```python
from build123d import *

# Parameters (mm, degrees)
SKETCH2_W           = 230
SKETCH2_H           = 200
BOSS_EXTRUDE1_DEPTH = 180
CUT_EXTRUDE1_DEPTH  = 200
FILLET2_R           = 40
SKETCH4_R           = 30
CUT_EXTRUDE2_DEPTH  = 48
SKETCH5_W           = 80
SKETCH5_H           = 129.575317766
CUT_EXTRUDE3_DEPTH  = 180
SKETCH6_R           = 15
CUT_EXTRUDE5_DEPTH  = 200


with BuildPart() as part:
    # Sketch2 → Boss-Extrude1 (new body)
    with BuildSketch(Plane(origin=(0, 0, 0), x_dir=(1, 0, 0), z_dir=(0, 1, 0))):
        with Locations((71.865714122, -63.208991457)):
            Rectangle(SKETCH2_W, SKETCH2_H)
    extrude(amount=BOSS_EXTRUDE1_DEPTH)

    # Sketch3 → Cut-Extrude1 (cut)
    with BuildSketch(Plane.XY.offset(163.208991457)):
        Polygon((100.422581047, 180), (186.865714122, 180), (186.865714122, 50.424682234), align=None)
    extrude(amount=-CUT_EXTRUDE1_DEPTH, mode=Mode.SUBTRACT)

    # Fillet2
    fillet2_edges = [part.edges().sort_by_distance(p)[0] for p in [
        (100.422581047, 180, 63.208991457),
        (-43.134285878, 180, 63.208991457),
    ]]
    fillet(fillet2_edges, radius=FILLET2_R)

    # Sketch4 → Cut-Extrude2 (cut)
    with BuildSketch(Plane.XZ):
        with Locations(Location((71.865714122, 63.208991457, 0), (0, 0, 270))):
            Circle(SKETCH4_R)
    extrude(amount=-CUT_EXTRUDE2_DEPTH, mode=Mode.SUBTRACT)

    # Sketch5 → Cut-Extrude3 (cut)
    with BuildSketch(Plane(origin=(186.865714122, 0, 0), x_dir=(0, 0, -1), z_dir=(1, 0, 0))):
        with Locations((-63.208991457, 115.212341117)):
            Rectangle(SKETCH5_W, SKETCH5_H)
    extrude(amount=-CUT_EXTRUDE3_DEPTH, mode=Mode.SUBTRACT)

    # Sketch6 → Cut-Extrude5 (cut)
    with BuildSketch(Plane.XY.offset(163.208991457)):
        with Locations((79.023419486, 140)):
            Circle(SKETCH6_R)
    extrude(amount=-CUT_EXTRUDE5_DEPTH, mode=Mode.SUBTRACT)


solid = part.part
```
Work out the finished part from the listing and answer in its coordinate system (mm). A direction names the side the tool comes from. Give positions to 0.01 mm unless a question says otherwise; leave off trailing zeros. Write each loop counter-clockwise with the first axis right and the second up, starting at its lowest first coordinate (ties: lowest second). Pieces come first, ordered by that corner, then holes.
(1) The part is cut by section D-D on x = 67. Write down the section's boundary in (y, z), plus the area to 3 significant figures.
Final values:
outline: (0, -36.79) - (131.03, -36.79) - (131.03, 23.21) - (50.42, 23.21) - (50.42, 103.21) - (131.03, 103.21) - (131.03, 163.21) - (0, 163.21) - (0, 92.81) - (48, 92.81) - (48, 33.61) - (0, 33.61) - close; (148.97, -36.79) - (180, -36.79) - (180, 23.21) - (148.97, 23.21) - close; (148.97, 103.21) - (180, 103.21) - (180, 163.21) - (148.97, 163.21) - close
area: 20,600 mm2
(2) The mould has two halves that part along Z. Classify faces 4 (the flat face through (45, 0, 40)), 5 (the flat face through (6.866, 116, 64)), 6 (the flat face through (70, 69, 163.209)): pulls with the +Z half, pulls with the -Z half, needs draft (parallel to the pull), parting line crosses it, or undercut.
Final values:
face 4: needs draft
face 5: undercut
face 6: pulls with the +Z half
(3) The part is cut by section A-A on y = 151.5. Write down the section's boundary in (x, z), plus the area to 3 significant figures.
Final values:
outline: (-41.45, -36.79) - (69.39, -36.79) - (69.39, 23.21) - (6.87, 23.21) - (6.87, 103.21) - (69.39, 103.21) - (69.39, 163.21) - (-41.45, 163.21) - close; (88.65, -36.79) - (119.44, -36.79) - (119.44, 23.21) - (88.65, 23.21) - close; (88.65, 103.21) - (119.44, 103.21) - (119.44, 163.21) - (88.65, 163.21) - close
area: 20,900 mm2
(4) Straight lines are drawn through the part: line 1 (Z direction, x = 37.5, y = 58.5); line 2 (X direction, y = 15, z = 61.5); line 3 (Y direction, x = 136, z = 97.5). For each, find the intervals that lie inside material, in ascending order.
Final values:
line 1: z = -36.79 to 23.21, 103.21 to 163.21
line 2: x = -43.13 to 41.91, 101.82 to 186.87
line 3: y = 0 to 50.42
(5) Which of the six approach directions +Z, -Z, +X, -X, +Y, -Y give full straight-line access (tool end or side, diameter ignored) to faces 1 (the cylindrical face through (-31.7, 168, 61.8)), 2 (the flat face through (72, 48, 64)), 3 (the flat face through (78, 100, 23.209))?
Final values:
face 1: +Z, -Z, -X, +Y
face 2: -Y
face 3: +X, +Y
(6) The part is cut by section C-C on x = 38.5. Write down the section's boundary in (y, z), plus the area to 3 significant figures.
Final values:
outline: (0, -36.79) - (180, -36.79) - (180, 23.21) - (50.42, 23.21) - (50.42, 103.21) - (180, 103.21) - (180, 163.21) - (0, 163.21) - close
area: 25,600 mm2
(7) Flat-ended cylindrical pins translate along their axes: pin 1 Ø10 at (x, z) = (141, 57) entering from +Y; pin 2 Ø12 at (y, z) = (87.5, 6.5) entering from +X; pin 3 Ø24 at (x, y) = (79.02, 140) entering from +Z; pin 4 Ø1.5 at (x, z) = (144.5, -5) entering from -Y. Find the tip coordinate at first contact, or state that the pin passes through.
Final values:
pin 1: stops at y = 50.42
pin 2: stops at x = 166.13
pin 3: passes through
pin 4: stops at y = 0
(8) The part is cut by section B-B on z = -10. Write down the section's boundary in (x, y).
Final values:
outline: (-43.13, 0) - (186.87, 0) - (186.87, 50.42) - (112.3, 162.2) arc R40 ccw to (79.02, 180) - (-3.13, 180) arc R40 ccw to (-43.13, 140) - close; hole circle Ø30 at (79.02, 140)
